Here's how the part is built. I have some questions about the finished solid (model axes, mm). Face numbers are marked on the shaded views. Coordinates: 2 decimals unless noted, no trailing zeros. Loops run counter-clockwise (first coordinate to the right, second up) from the corner with the lowest first, then second, coordinate; pieces in that order, holes last. Notation, with made-up numbers: (10, -35.5) -> (62, -35.5) arc R19 ccw to (62, -4.5) -> close; hole circle Ø7 at (28, 36). An arc over 180 degrees is marked (long way). Answer as a JSON object with one key per item and string values. Group by question number.
Q1. I need wall thicknesses on line 1 (Y direction, x = 12.5, z = 0); line 2 (Z direction, x = 5.25, y = -4.5); line 3 (Y direction, x = 1.75, z = 5). Which ranges of each line are inside material? Lowest first, please.
Q2. Thinking about a two-plate mould opening in Z: for the marked faces 1, 2 and 3, which applies, released by +Z, released by -Z, zero draft, split by the parting line, or undercut?
Q3. I want a section at C-C on x = 12. Write out the boundary of the cut face in (y, z), then the cut area to 3 significant figures.
Q4. I'm going to push flat-ended pins straight in: pin 1 (16.5 mm diameter, centred on y = 0, z = 0, fed in from -X); pin 2 (4 mm diameter, centred on x = 5, z = 6, fed in from +Y); pin 3 (3 mm diameter, centred on x = 9.5, y = -9.5, fed in from -Z); pin 4 (1.5 mm diameter, centred on x = 5.5, y = -6, fed in from +Z). Where does each tip first touch, or does it pass through?
Q5. I want a section at A-A on z = 0. Write out the boundary of the cut face in (x, y).
```python
from build123d import *

# Parameters (mm, degrees)
SKETCH2_R           = 25.4
BOSS_EXTRUDE1_DEPTH = 25.4
FILLET1_R           = 6.35
SKETCH3_R           = 6.35
CUT_EXTRUDE1_DEPTH  = 25.4


with BuildPart() as part:
    # Sketch2 → Boss-Extrude1 (new body)
    with BuildSketch(Plane(origin=(0, 0, 0), x_dir=(0, 0, -1), z_dir=(1, 0, 0))):
        Circle(SKETCH2_R)
    extrude(amount=BOSS_EXTRUDE1_DEPTH)

    # Fillet1
    fillet1_edges = [part.edges().sort_by_distance(p)[0] for p in [
        (0, 0, 25.4),
        (25.4, 0, 25.4),
    ]]
    fillet(fillet1_edges, radius=FILLET1_R)

    # Sketch3 → Cut-Extrude1 (cut)
    with BuildSketch(Plane(origin=(25.4, 0, 0), x_dir=(0, 0, -1), z_dir=(1, 0, 0))):
        Circle(SKETCH3_R)
    extrude(amount=-CUT_EXTRUDE1_DEPTH, mode=Mode.SUBTRACT)


solid = part.part
```
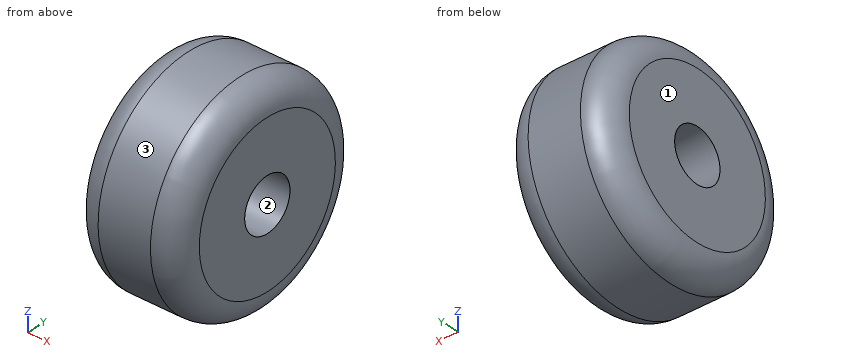
Result set:
{
 "1": {"line 1": "y = -25.4 to -6.35, 6.35 to 25.4", "line 2": "z = -24.9 to -4.48, 4.48 to 24.9", "line 3": "y = -22.89 to -3.91, 3.91 to 22.89"},
 "2": {"face 1": "zero draft", "face 2": "undercut", "face 3": "split by the parting line"},
 "3": {"outline": "circle Ø50.8 at (0, 0); hole circle Ø12.7 at (0, 0)", "area": "1,900 mm²"},
 "4": {"pin 1": "stops at x = 0", "pin 2": "stops at y = 25.03", "pin 3": "stops at z = -24.11", "pin 4": "stops at z = 24.81"},
 "5": {"outline": "(0, -19.05) arc R6.35 ccw to (6.35, -25.4) -> (19.05, -25.4) arc R6.35 ccw to (25.4, -19.05) -> (25.4, -6.35) -> (0, -6.35) -> close; (0, 6.35) -> (25.4, 6.35) -> (25.4, 19.05) arc R6.35 ccw to (19.05, 25.4) -> (6.35, 25.4) arc R6.35 ccw to (0, 19.05) -> close"}
}
